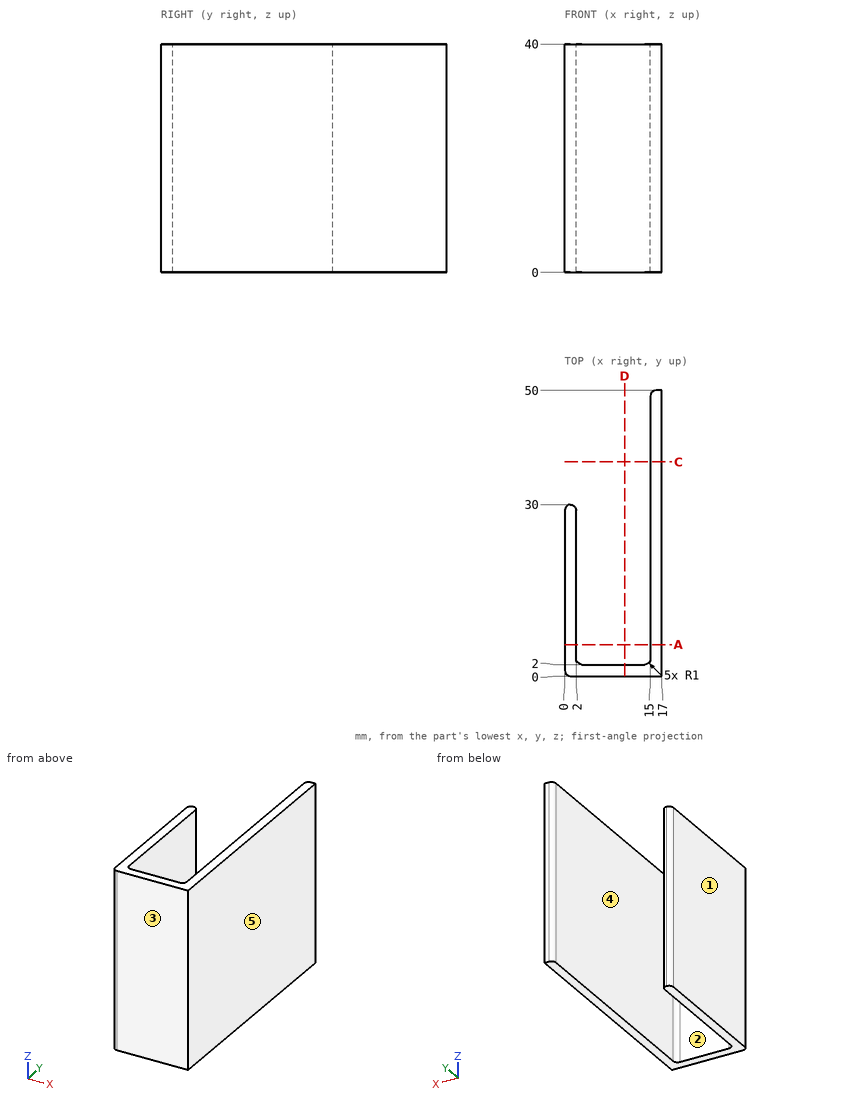
The drawing under review shows one solid part. Ordinate dimensions are in mm from its lowest x, y, z. A direction names the side the tool comes from. Coordinates: 2 decimals unless noted, no trailing zeros. Write each loop counter-clockwise with the first axis right and the second up, starting at its lowest first coordinate (ties: lowest second). Pieces come first, ordered by that corner, then holes. Notation, with made-up numbers: (58.5, 54.5) - (73.5, 54.5) arc R14 ccw to (73.5, 59.5) - close; hole circle Ø9 at (83.25, -18.75). An arc over 180 degrees is marked (long way). Answer in a Markdown table with one row per item. Add a question column.
Q1. Draft analysis for pull direction X (two halves, no side actions). For the marked faces 3, 4 and 5, state which applies: +X half, -X half, draft (parallel to the pull), parting line (faces both ways), or undercut.
Q2. Tool access review of the marked faces 1 and 2: name each direction out of +Z, -Z, +X, -X, +Y, -Y from which nothing blocks a thin tool from reaching the whole face with its end or side.
Q3. We need section D-D, the plane x = 10.5. State the section outline as (y, z) points.
Q4. We need section C-C, the plane y = 37.5. State the section outline as (x, z) points, and give its area (3 significant figures).
Q5. For P1, Ø9, axis at x = 8, z = 24.5, coming from the +Y side; P2, Ø12, axis at y = 21, z = 12, coming from the -X side; P3, Ø8, axis at x = 5, z = 14.5, coming from the +Y side, all flat-tipped, find the tip position at first contact; note any pin that passes through.
Q6. We need section A-A, the plane y = 5.5. State the section outline as (x, z) points.
Q7. For probe 1 along X at (y, z) = (9, 28); probe 2 along Y at (x, z) = (13.5, 4); probe 3 along X at (y, z) = (37, 34.5), list the stretches that pass through material, from the lowest coordinate up.
Answer list:
| question | item | result |
|---|---|---|
| 1 | face 3 | draft |
| 1 | face 4 | undercut |
| 1 | face 5 | +X half |
| 2 | face 1 | +Z, -Z, -X, +Y, -Y |
| 2 | face 2 | +Z, -Z, +Y |
| 3 | outline | (0, 0) - (2, 0) - (2, 40) - (0, 40) - close |
| 4 | outline | (15, 0) - (17, 0) - (17, 40) - (15, 40) - close |
| 4 | area | 80.0 mm2 |
| 5 | P1 | stops at y = 2 |
| 5 | P2 | stops at x = 0 |
| 5 | P3 | stops at y = 30 |
| 6 | outline | (0, 0) - (2, 0) - (2, 40) - (0, 40) - close; (15, 0) - (17, 0) - (17, 40) - (15, 40) - close |
| 7 | probe 1 | x = 0 to 2, 15 to 17 |
| 7 | probe 2 | y = 0 to 2 |
| 7 | probe 3 | x = 15 to 17 |
